Source: CAD feature listing. Evaluate the final solid. Frame: model axes, mm. Round coordinates to 2 decimals unless told otherwise and drop trailing zeros. Write each loop counter-clockwise with the first axis right and the second up, starting at its lowest first coordinate (ties: lowest second). Pieces come first, ordered by that corner, then holes.
from build123d import *

# Parameters (mm, degrees)
SKETCH2_W           = 203.2
SKETCH2_H           = 25.4
BOSS_EXTRUDE1_DEPTH = 12.7
SKETCH13_R          = 1.27
CUT_EXTRUDE2_DEPTH  = 207.350575478
SKETCH16_R          = 1.905
CUT_EXTRUDE4_DEPTH  = 207.350575478


with BuildPart() as part:
    # Sketch2 → Boss-Extrude1 (new, symmetric)
    with BuildSketch(Plane.XY):
        with Locations((101.6, 12.7)):
            Rectangle(SKETCH2_W, SKETCH2_H)
    extrude(amount=BOSS_EXTRUDE1_DEPTH, both=True)

    # Sketch13 → Cut-Extrude2 (cut, through all)
    with BuildSketch(Plane.XY.offset(12.7)):
        with Locations((165.1, 12.7)):
            Circle(SKETCH13_R)
        with Locations((184.15, 12.7)):
            Circle(SKETCH13_R)
        with Locations((171.425836333, 13.253438966)):
            Circle(SKETCH13_R)
        with Locations((177.676404473, 14.467498382)):
            Circle(SKETCH13_R)
    extrude(amount=-CUT_EXTRUDE2_DEPTH, mode=Mode.SUBTRACT)

    # Sketch18 → Cut-Revolve2 (revolve, cut)
    with BuildSketch(Plane.XY, mode=Mode.PRIVATE) as cut_revolve2_sk:
        Polygon((152.4, 25.4), (153.67, 25.4), (153.67, 15.24), (152.4, 13.040295474), align=None)
    cut_revolve2 = revolve(cut_revolve2_sk.sketch.rotate(Axis((152.4, 13.040295474, 0), (0, 1, 0)), 90), axis=Axis((152.4, 13.040295474, 0), (0, 1, 0)), mode=Mode.SUBTRACT)

    # Mirror2: Cut-Revolve2 across plane
    add(cut_revolve2.mirror(Plane(origin=(155.575, 0, 0), x_dir=(0, 0, 1), z_dir=(1, 0, 0))), mode=Mode.SUBTRACT)

    # Sketch16 → Cut-Extrude4 (cut, through all)
    with BuildSketch(Plane.XY.offset(12.7)):
        with Locations((50.8, 13.625917973)):
            Circle(SKETCH16_R)
        with Locations((66.04, 13.625917973)):
            Circle(SKETCH16_R)
    extrude(amount=-CUT_EXTRUDE4_DEPTH, mode=Mode.SUBTRACT)


solid = part.part
1) Section query A-A on x = 50.8. Return the cut outline in (y, z).
Taken from the geometry:
outline: (0, -12.7) - (11.72, -12.7) - (11.72, 12.7) - (0, 12.7) - close; (15.53, -12.7) - (25.4, -12.7) - (25.4, 12.7) - (15.53, 12.7) - close
2) Contact query for a flat-ended pin moving along its axis: P1, Ø3.5, axis at x = 66.04, y = 13.63, coming from the -Z side. Output: stop coordinate, or through.
Taken from the geometry:
P1: passes through
3) Material intervals for line 1 (X direction, y = 18.25, z = 0); line 2 (Y direction, x = 184.15, z = 5.25); line 3 (Y direction, x = 66.04, z = -5.75), sorted ascending.
Taken from the geometry:
line 1: x = 0 to 151.13, 153.67 to 157.48, 160.02 to 203.2
line 2: y = 0 to 11.43, 13.97 to 25.4
line 3: y = 0 to 11.72, 15.53 to 25.4
4) Pull-direction query (Y, two-part tool) for faces 1 (the face through (100, 0, 0)), 2 (the face through (67.8, 12.9, 0.2)), 3 (the face through (100, 13, 12.7)); classes: released by +Y, released by -Y, zero draft, split by the parting line, or undercut.
Taken from the geometry:
face 1: released by -Y
face 2: undercut
face 3: zero draft
